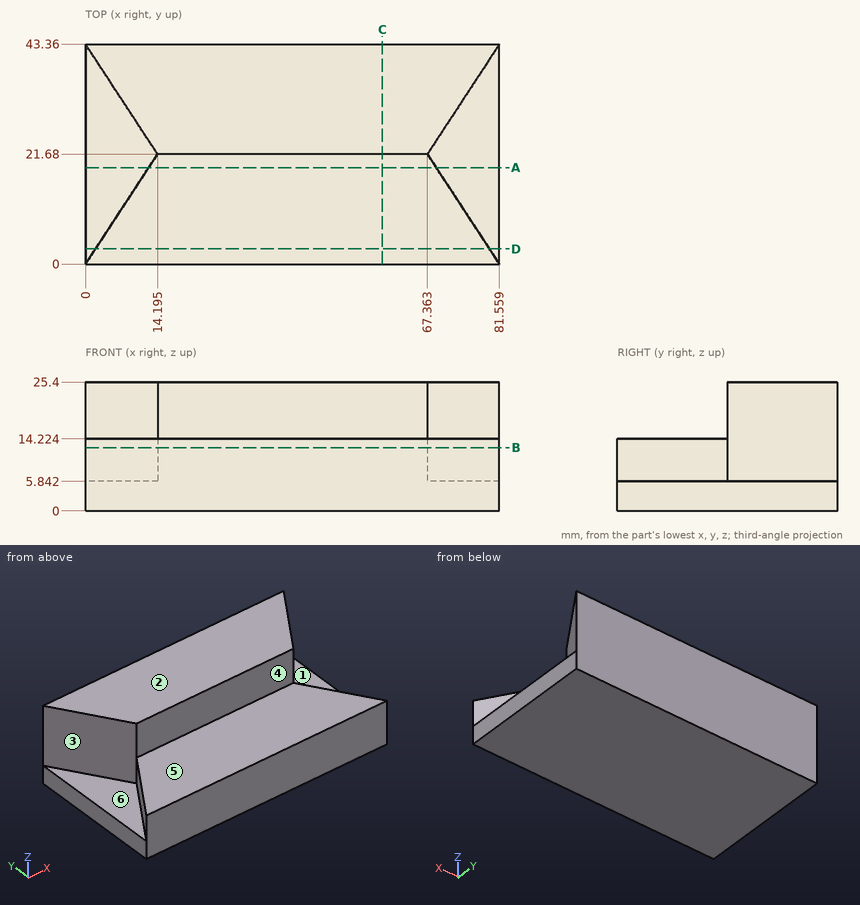
Verification items for this drawing (mm, ordinates from the low corner). A direction names the side the tool comes from. Coordinates: 2 decimals unless noted, no trailing zeros. Write each loop counter-clockwise with the first axis right and the second up, starting at its lowest first coordinate (ties: lowest second). Pieces come first, ordered by that corner, then holes. Notation, with made-up numbers: M 48,71.25 L 53,71.25 A11 ccw 53,82.25 Z; hole C -9,45 d3. An arc over 180 degrees is marked long. One line per item, written item: value. Start each with the question number.
(1) Sectioned sample at D-D, the plane y = 3. Enter the section's corners in (x, z) (1 decimal), and give its area (3 significant figures).
(2) Scan lines: line 1 along Z through (x, y) = (19.5, 5); line 2 along Z through (x, y) = (72.5, 24); line 3 along Y through (x, z) = (23, 15). Record each from-to range of solid material in increasing order. Write a range as [from, to].
(3) Sectioned sample at C-C, the plane x = 58.5. Enter the section's corners in (y, z), and give its area (3 significant figures).
(4) Tool access check on the marked faces 1 and 2. Record the directions out of +Z, -Z, +X, -X, +Y, -Y that give a thin tool (end or side, any length) a straight path to the whole face; none if there is none.
(5) Sectioned sample at B-B, the plane z = 12.5. Enter the section's corners in (x, y) (1 decimal), and give its area (3 significant figures).
(6) Sectioned sample at A-A, the plane y = 19. Enter the section's corners in (x, z).
(7) Release check for a two-part mould opening along Y. For the marked faces 3, 4, 5 and 6 record: released by +Y, released by -Y, zero draft, split by the parting line, or undercut.
(8) Depth check by flat-ended pin: pin 1 (9 mm diameter, centred on x = 53, z = 19.5, fed in from -Y); pin 2 (11.5 mm diameter, centred on x = 77.5, y = 17, fed in from +Z); pin 3 (1.5 mm diameter, centred on y = 7.5, z = 12.5, fed in from +X). Enter the tip coordinate at first touch or a pass-through.
Filled sheet:
1. outline: M 0,0 L 81.6,0 L 81.6,5.8 L 79.6,5.8 L 79.6,14.2 L 2,14.2 L 2,5.8 L 0,5.8 Z
1. area: 1,130 mm²
2. line 1: [0, 14.22]
2. line 2: [0, 5.84]
2. line 3: [21.68, 43.36]
3. outline: M 0,0 L 43.36,0 L 43.36,25.4 L 21.68,25.4 L 21.68,14.22 L 0,14.22 Z
3. area: 859 mm²
4. face 1: +Z, +X
4. face 2: +Z, +X, -X, +Y, -Y
5. outline: M 0,0 L 81.6,0 L 67.4,21.7 L 81.6,43.4 L 0,43.4 L 14.2,21.7 Z
5. area: 2,920 mm²
6. outline: M 0,0 L 81.56,0 L 81.56,5.84 L 69.12,5.84 L 69.12,14.22 L 12.44,14.22 L 12.44,5.84 L 0,5.84 Z
7. face 3: undercut
7. face 4: released by -Y
7. face 5: zero draft
7. face 6: undercut
8. pin 1: y = 21.68
8. pin 2: z = 5.84
8. pin 3: x = 77.14
